```python
from build123d import *

# Parameters (mm, degrees)
F1_R     = 6
F2_DEPTH = 240


with BuildPart() as f2:
    # F1 (on Front) → F2 (new body, symmetric)
    with BuildSketch(Plane.XZ):
        Circle(F1_R)
    extrude(amount=F2_DEPTH, both=True)


with BuildPart() as f3_1:
    # F3: copy of F2
    add(f2.part)


solid = f2.part
```
Check sheet for the modelled part. Datum: model origin and axes. Units: mm. Coordinates: 2 decimals unless noted, no trailing zeros. Write each loop counter-clockwise with the first axis right and the second up, starting at its lowest first coordinate (ties: lowest second). Pieces come first, ordered by that corner, then holes. Notation, with made-up numbers: (63.5, 33) -> (109.5, 33) arc R4 ccw to (109.5, 37) -> close; hole circle Ø1 at (-27.75, -18). An arc over 180 degrees is marked (long way). Use a Markdown table: item, result.
1. Sectioned sample at C-C (z = -2.5). Enter the section's corners in (x, y).
Reported:
| item | result |
|---|---|
| outline | (-5.45, -240) -> (5.45, -240) -> (5.45, 240) -> (-5.45, 240) -> close |
2. Sectioned sample at B-B (x = 1.25). Enter the section's corners in (y, z), plus the area to 3 significant figures.
Reported:
| item | result |
|---|---|
| outline | (-240, -5.87) -> (240, -5.87) -> (240, 5.87) -> (-240, 5.87) -> close |
| area | 5,630 mm2 |
3. Go/stop test with flat-tipped pins: pin 1 Ø6 at (y, z) = (51.5, -4.5) entering from +X; pin 2 Ø5 at (x, y) = (-1, -15.5) entering from +Z; pin 3 Ø1.5 at (y, z) = (41, 3.5) entering from +X. Record where each tip stops, or that it passes through.
Reported:
| item | result |
|---|---|
| pin 1 | stops at x = 5.81 |
| pin 2 | stops at z = 6 |
| pin 3 | stops at x = 5.33 |
4. Sectioned sample at A-A (y = 200). Enter the section's corners in (x, z), plus the area to 3 significant figures.
Reported:
| item | result |
|---|---|
| outline | circle Ø12 at (0, 0) |
| area | 113 mm2 |
5. Scan lines: line 1 along X through (y, z) = (56.5, 0.75); line 2 along Z through (x, y) = (1, 54). Record each from-to range of solid material in increasing order.
Reported:
| item | result |
|---|---|
| line 1 | x = -5.95 to 5.95 |
| line 2 | z = -5.92 to 5.92 |
